Check sheet for the modelled part. Datum: model origin and axes. Units: mm. A direction names the side the tool comes from. Give positions to 0.01 mm unless a question says otherwise; leave off trailing zeros. Order: outer loops, then holes, each group sorted by start corner. A loop starts at its lowest first (then second) coordinate and runs counter-clockwise, first axis right, second up.
```python
from build123d import *

# Parameters (mm, degrees)
SKETCH_1_R          = 30
SKETCH_1_R_2        = 19
EXTRUDE_1_DEPTH     = 55
CUT_EXTRUDE_1_DEPTH = 70.462219947
SKETCH_3_R          = 33.5
SKETCH_3_R_2        = 27.5
EXTRUDE_2_DEPTH     = 10
SKETCH_4_R          = 2.5
CUT_EXTRUDE_2_DEPTH = 34
CHAMFER_1_SIZE      = 0.5


with BuildPart() as part:
    # 草图1 → 拉伸1 (new body)
    with BuildSketch(Plane.XY):
        Circle(SKETCH_1_R)
        Circle(SKETCH_1_R_2, mode=Mode.SUBTRACT)
    extrude(amount=EXTRUDE_1_DEPTH)

    # 草图2 → 切除-拉伸1 (cut, through all)
    with BuildSketch(Plane.XY.offset(55)):
        with BuildLine():
            Line((5, 19), (5, 18.33030278))
            ThreePointArc((5, 18.33030278), (0, 19), (-5, 18.33030278))
            Line((-5, 18.33030278), (-5, 19))
            Line((-5, 19), (-5, 22))
            Line((-5, 22), (5, 22))
            Line((5, 22), (5, 19))
        make_face()
    extrude(amount=-CUT_EXTRUDE_1_DEPTH, mode=Mode.SUBTRACT)

    # 草图3 → 拉伸2 (add)
    with BuildSketch(Plane.XY.offset(55)):
        Circle(SKETCH_3_R)
        Circle(SKETCH_3_R_2, mode=Mode.SUBTRACT)
    extrude(amount=-EXTRUDE_2_DEPTH)

    # 草图4 → 切除-拉伸2 (cut)
    with BuildSketch(Plane(origin=(0, 0, 0), x_dir=(-1, 0, 0), z_dir=(0, 0, -1))):
        with Locations(Location((12.5, 21.650635095, 0), (0, 0, 90))):
            Circle(SKETCH_4_R)
        with Locations(Location((25, 0, 0), (0, 0, 90))):
            Circle(SKETCH_4_R)
        with Locations(Location((12.5, -21.650635095, 0), (0, 0, 90))):
            Circle(SKETCH_4_R)
        with Locations(Location((-12.5, -21.650635095, 0), (0, 0, 90))):
            Circle(SKETCH_4_R)
        with Locations(Location((-25, 0, 0), (0, 0, 90))):
            Circle(SKETCH_4_R)
        with Locations(Location((-12.5, 21.650635095, 0), (0, 0, 90))):
            Circle(SKETCH_4_R)
    extrude(amount=-CUT_EXTRUDE_2_DEPTH, mode=Mode.SUBTRACT)

    # 倒角1
    chamfer_1_edges = [part.edges().sort_by_distance(p)[0] for p in [
        (0, -19, 0),
        (-30, 0, 0),
        (-33.5, 0, 55),
        (-33.5, 0, 45),
        (0, -19, 55),
    ]]
    chamfer(chamfer_1_edges, length=CHAMFER_1_SIZE)


solid = part.part
```
(1) Cross-section at C-C on x = 0. Enter the section's corners in (y, z), then the cut area to 3 significant figures.
Response values:
outline: (-33.5, 45.5) - (-33, 45) - (-30, 45) - (-30, 0.5) - (-29.5, 0) - (-19.5, 0) - (-19, 0.5) - (-19, 54.5) - (-19.5, 55) - (-33, 55) - (-33.5, 54.5) - close; (22, 0) - (29.5, 0) - (30, 0.5) - (30, 45) - (33, 45) - (33.5, 45.5) - (33.5, 54.5) - (33, 55) - (22, 55) - close
area: 1,110 mm2
(2) Material ranges on L1, parallel to X at y = 0, z = 18; L2, parallel to Y at x = 0, z = 40; L3, parallel to X at y = 0, z = 37, recorded low to high.
Response values:
L1: x = -30 to -27.5, -22.5 to -19, 19 to 22.5, 27.5 to 30
L2: y = -30 to -19, 22 to 30
L3: x = -30 to -19, 19 to 30
(3) Gauge pin test, flat ends, axial feed: pin 1 Ø4 at (y, z) = (21, 21.5) entering from +X; pin 2 Ø4 at (y, z) = (-1.5, 16.5) entering from -X; pin 3 Ø8 at (y, z) = (17, 25.5) entering from +X; pin 4 Ø8 at (x, y) = (-6.5, -9) entering from -Z. Record the tip position at first contact, or that the pin passes through.
Response values:
pin 1: stops at x = 23.22
pin 2: stops at x = -30
pin 3: stops at x = 27.04
pin 4: passes through
(4) Cross-section at B-B on z = 39. Enter the section's corners in (x, y), then the cut area to 3 significant figures.
Response values:
outline: circle Ø60 at (0, 0); hole (-5, 18.33) arc R19 ccw (long way) to (5, 18.33) - (5, 22) - (-5, 22) - close
area: 1,660 mm2
(5) Release check for a two-part mould opening along Y. For faces 4 (the face through (27.48, -0.33, 16.76)), 5 (the face through (-7.262, -32.703, 50.063)), 6 (the face through (14, -14, 55)) record: released by +Y, released by -Y, zero draft, split by the parting line, or undercut.
Response values:
face 4: undercut
face 5: split by the parting line
face 6: zero draft
(6) Set-up check for faces 1 (the face through (0.772, -19.12, 54.635)), 2 (the face through (10.28, 22.8, 16.76)), 3 (the face through (5, 20, 28)): record each of +Z, -Z, +X, -X, +Y, -Y from which the full face is reachable in a straight line by a thin tool's end or side.
Response values:
face 1: +Z
face 2: -Z
face 3: +Z, -Z
(7) Cross-section at D-D on z = 27.5. Enter the section's corners in (x, y).
Response values:
outline: circle Ø60 at (0, 0); hole circle Ø5 at (-25, 0); hole circle Ø5 at (-12.5, -21.65); hole circle Ø5 at (-12.5, 21.65); hole (-5, 18.33) arc R19 ccw (long way) to (5, 18.33) - (5, 22) - (-5, 22) - close; hole circle Ø5 at (12.5, -21.65); hole circle Ø5 at (12.5, 21.65); hole circle Ø5 at (25, 0)
